Input: dimensioned drawing with shaded views. Units: mm. Origin: part minimum x, y, z. Give positions to 0.01 mm unless a question says otherwise; leave off trailing zeros. Loops run counter-clockwise (first coordinate to the right, second up) from the corner with the lowest first, then second, coordinate; pieces in that order, holes last.
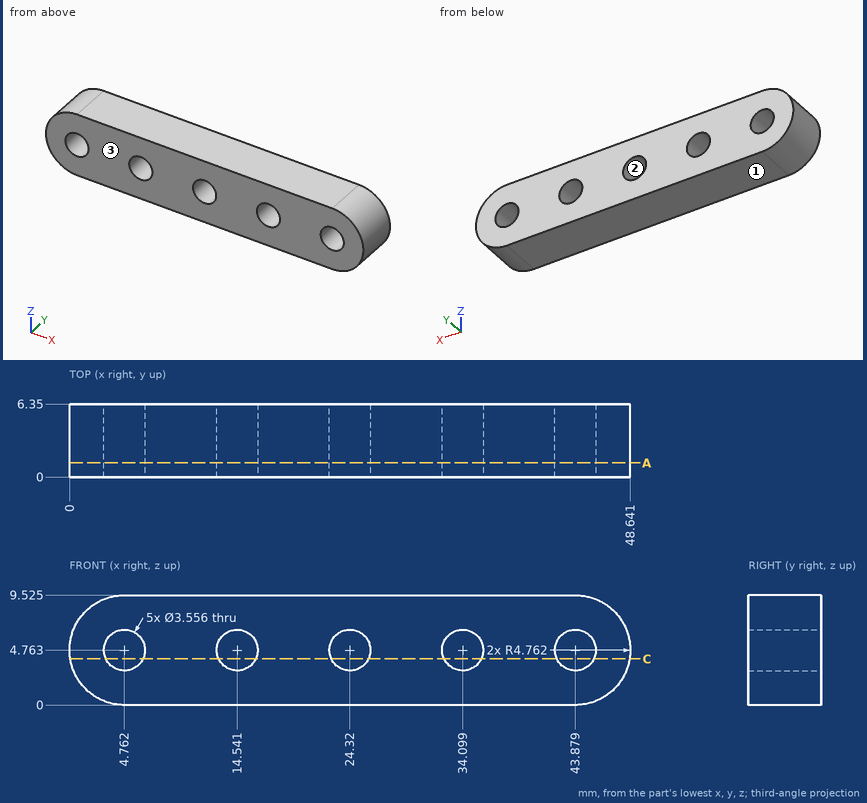
Item 1: Draft query along Z for the marked faces 1, 2 and 3. Return one class per face: +Z half, -Z half, draft (parallel to the pull), parting line (faces both ways), or undercut.
Values follow:
face 1: -Z half
face 2: undercut
face 3: draft
Item 2: Section query C-C on z = 4. Give the number of separate pieces and of enclosed holes in the cut face, plus the area to 3 significant figures.
Values follow:
separate pieces: 6
enclosed holes: 0
area: 206 mm2
Item 3: Section query A-A on y = 1.25. Return loops of the section in (x, z) (1 decimal).
Values follow:
outline: (4.8, 0) - (43.9, 0) arc R4.8 ccw to (43.9, 9.5) - (4.8, 9.5) arc R4.8 ccw to start; hole circle Ø3.6 at (4.8, 4.8); hole circle Ø3.6 at (14.5, 4.8); hole circle Ø3.6 at (24.3, 4.8); hole circle Ø3.6 at (34.1, 4.8); hole circle Ø3.6 at (43.9, 4.8)
Item 4: Pin query (flat end, axial travel): pin 1 (4.5 mm diameter, centred on x = 14.54, z = 4.76, fed in from +Y); pin 2 (3 mm diameter, centred on x = 34.1, z = 4.76, fed in from -Y); pin 3 (1 mm diameter, centred on y = 3.5, z = 2.5, fed in from +X). Return the tip coordinate at first contact, or that it passes through.
Values follow:
pin 1: stops at y = 6.35
pin 2: passes through
pin 3: stops at x = 48.3
Item 5: Ray query, probe 1 along Z at (x, y) = (44, 4.75); probe 2 along X at (y, z) = (3.5, 4.25) (1 decimal); probe 3 along X at (y, z) = (5.75, 6) (1 decimal). Return the intervals inside material, ascending.
Values follow:
probe 1: z = 0 to 2.99, 6.54 to 9.52
probe 2: x = 0 to 3.1, 6.5 to 12.8, 16.2 to 22.6, 26 to 32.4, 35.8 to 42.2, 45.6 to 48.6
probe 3: x = 0.2 to 3.5, 6 to 13.3, 15.8 to 23, 25.6 to 32.8, 35.4 to 42.6, 45.2 to 48.5
